Design review of the part built by this model. Coordinates are the model's own, in mm. A direction names the side the tool comes from. Round coordinates to 2 decimals unless told otherwise and drop trailing zeros. Order: outer loops, then holes, each group sorted by start corner. A loop starts at its lowest first (then second) coordinate and runs counter-clockwise, first axis right, second up. Notation, with made-up numbers: M 60,76.5 L 103,76.5 A29 cw 103,97.5 Z; hole C -20,40 d1. An arc over 180 degrees is marked long. Use a Markdown table: item, result. Add a question column.
(1) Machinability: for faces 4 (the face through (22, -17.2, 1)), 5 (the face through (-13.417, -29.187, 1.014)), 6 (the face through (17, -22.1, 1)), 7 (the face through (28.733, 5.205, 1.014)), 8 (the face through (-25, 25, 1)), which of the approach directions +Z, -Z, +X, -X, +Y, -Y give a long, thin tool a straight path to every point of the face, cutting with its end or side? Answer none if there is none.
(2) Take a section at C-C (x = -28.5). Write out the cut boundary in (y, z).
(3) Take a section at B-B (z = 1.3). Write out the cut boundary in (x, y), then the cut area to 3 significant figures.
(4) Take a section at A-A (y = 21.73). Write out the cut boundary in (x, z).
(5) Take a section at D-D (y = -8.6). Write out the cut boundary in (x, z), then the cut area to 3 significant figures.
(6) The part is to be moulded in two halves that separate along Y. For faces 1 (the face through (-28.733, 5.205, 1.014)), 2 (the face through (-17, -22.1, 1)), 3 (the face through (32.364, -4, 1)), say which applies: released by +Y, released by -Y, zero draft, split by the parting line, or undercut.
(7) To check wall thickness, follow probe 1 along X at (y, z) = (15.5, 1.9); probe 2 along Y at (x, z) = (-28.5, 0.95); probe 3 along Y at (x, z) = (19.5, 0.3). State the ranges of each line that lie inside material, in increasing order. Write a range as from..to.
```python
from build123d import *

# Parameters (mm, degrees)
EXTRUDE1_DEPTH  = 2
SKETCH4_R       = 1.5
EXTRUDE3_DEPTH  = 2
EXTRUDE5_DEPTH  = 2
FILLET2_R       = 3
SKETCH7_R       = 1.5
EXTRUDE6_DEPTH  = 2
EXTRUDE7_DEPTH  = 2
EXTRUDE8_DEPTH  = 2
EXTRUDE9_DEPTH  = 2
EXTRUDE10_DEPTH = 2
EXTRUDE11_DEPTH = 2
SKETCH13_W      = 52.444820885
SKETCH13_H      = 24.426279397
EXTRUDE12_DEPTH = 2
SKETCH14_R      = 1.5
EXTRUDE13_DEPTH = 2


with BuildPart() as part:
    # Sketch1 → Extrude1 (new body)
    with BuildSketch(Plane.XY):
        Polygon((-15, 13.5), (-15, 38.5), (15, 38.5), (15, 13.5), (26.811651575, -4.688348425), (15, -16.5), (15, -26.5), (7.928932188, -33.571067812), (7.928932188, -52.571067812), (-7.928932188, -52.571067812), (-7.928932188, -33.571067812), (-15, -26.5), (-15, -16.5), (-26.811651575, -4.688348425), align=None)
    extrude(amount=EXTRUDE1_DEPTH)

    # Sketch4 → Extrude3 (add)
    with BuildSketch(Plane.XY.offset(2)):
        Polygon((-26.811651575, -4.688348425), (-32.363678884, -6.963209468), (-30.088817841, -12.515236776), (-22.212122569, -9.287877431), align=None)
        with Locations((-28.5, -8.6)):
            Circle(SKETCH4_R, mode=Mode.SUBTRACT)
    extrude3 = extrude(amount=-EXTRUDE3_DEPTH)

    # Mirror1: Extrude3 across plane
    add(extrude3.mirror(Plane(origin=(0, 0, 0), x_dir=(0, 0, 1), z_dir=(1, 0, 0))))

    # Sketch6 → Extrude5 (add)
    with BuildSketch(Plane.XY.offset(2)):
        Polygon((0, -44.571067812), (-7.928932188, -44.571067812), (-18, -54.642135624), (18, -54.642135624), (7.928932188, -44.571067812), align=None)
    extrude(amount=-EXTRUDE5_DEPTH)

    # Fillet2
    fillet2_edges = [part.edges().sort_by_distance(p)[0] for p in [
        (18, -54.642135624, 1),
        (-18, -54.642135624, 1),
    ]]
    fillet(fillet2_edges, radius=FILLET2_R)

    # Sketch7 → Extrude6 (cut)
    with BuildSketch(Plane.XY.offset(2)):
        with Locations((-11, -52.002135624)):
            Circle(SKETCH7_R)
    extrude6 = extrude(amount=-EXTRUDE6_DEPTH, mode=Mode.SUBTRACT)

    # Mirror4: Extrude6 across plane
    add(extrude6.mirror(Plane(origin=(0, 0, 0), x_dir=(0, 0, 1), z_dir=(1, 0, 0))), mode=Mode.SUBTRACT)

    # Sketch8 → Extrude7 (add)
    with BuildSketch(Plane.XY.offset(2)):
        Polygon((-26.811651575, -4.688348425), (-32.363678884, -6.963209468), (-32.363678884, -0.385171544), (-15, 26.352549211), (-15, 13.5), align=None)
    extrude7 = extrude(amount=-EXTRUDE7_DEPTH)

    # Sketch9 → Extrude8 (add)
    with BuildSketch(Plane.XY.offset(2)):
        Polygon((-22.212122569, -9.287877431), (-25.22165278, -10.520987907), (-15, -20.742640687), (-15, -16.5), align=None)
    extrude8 = extrude(amount=-EXTRUDE8_DEPTH)

    # Sketch10 → Extrude9 (add)
    with BuildSketch(Plane.XY.offset(2)):
        Polygon((-25.22165278, -10.520987907), (-30.088817841, -12.515236776), (-23.702612277, -18.90144234), (-20.271905312, -15.470735375), align=None)
    extrude9 = extrude(amount=-EXTRUDE9_DEPTH)

    # Sketch11 → Extrude10 (add)
    with BuildSketch(Plane.XY.offset(2)):
        Polygon((-15.322157844, -20.420482843), (-18.752864809, -23.851189808), (-7.928932188, -34.675122429), (-7.928932188, -33.571067812), (-15, -26.5), (-15, -20.742640687), align=None)
    extrude10 = extrude(amount=-EXTRUDE10_DEPTH)

    # Sketch12 → Extrude11 (add)
    with BuildSketch(Plane.XY.offset(2)):
        Polygon((-25, 10.953899573), (-25, 38.5), (-15, 38.5), (-15, 26.352549211), align=None)
    extrude11 = extrude(amount=-EXTRUDE11_DEPTH)

    # Mirror5: Extrude7, Extrude8, Extrude9, Extrude10 across plane
    add(extrude7.mirror(Plane(origin=(0, 0, 0), x_dir=(0, 0, 1), z_dir=(1, 0, 0))))
    add(extrude8.mirror(Plane(origin=(0, 0, 0), x_dir=(0, 0, 1), z_dir=(1, 0, 0))))
    add(extrude9.mirror(Plane(origin=(0, 0, 0), x_dir=(0, 0, 1), z_dir=(1, 0, 0))))
    add(extrude10.mirror(Plane(origin=(0, 0, 0), x_dir=(0, 0, 1), z_dir=(1, 0, 0))))

    # Mirror6: Extrude11 across plane
    add(extrude11.mirror(Plane(origin=(0, 0, 0), x_dir=(0, 0, 1), z_dir=(1, 0, 0))))

    # Sketch13 → Extrude12 (cut)
    with BuildSketch(Plane(origin=(0, 0, 0), x_dir=(-1, 0, 0), z_dir=(0, 0, -1))):
        with Locations((1.088066824, -46.888262128)):
            Rectangle(SKETCH13_W, SKETCH13_H)
    extrude(amount=-EXTRUDE12_DEPTH, mode=Mode.SUBTRACT)

    # Sketch14 → Extrude13 (cut)
    with BuildSketch(Plane.XY.offset(2)):
        with Locations((-20, 21.73)):
            Circle(SKETCH14_R)
        with Locations((20, 21.73)):
            Circle(SKETCH14_R)
    extrude(amount=-EXTRUDE13_DEPTH, mode=Mode.SUBTRACT)


solid = part.part
```
Verdict:
| question | item | result |
|---|---|---|
| 1 | face 4 | +Z, -Z, -Y |
| 1 | face 5 | +Z, -Z, -X, -Y |
| 1 | face 6 | +Z, -Z, +X |
| 1 | face 7 | +Z, -Z, +X, +Y |
| 1 | face 8 | +Z, -Z, -X, +Y |
| 2 | outline | M -14.1,0 L -10.1,0 L -10.1,2 L -14.1,2 Z; M -7.1,0 L 5.56,0 L 5.56,2 L -7.1,2 Z |
| 3 | outline | M -32.36,-6.96 L -30.09,-12.52 L -23.7,-18.9 L -20.27,-15.47 L -15.32,-20.42 L -18.75,-23.85 L -7.93,-34.68 L 7.93,-34.68 L 18.75,-23.85 L 15.32,-20.42 L 20.27,-15.47 L 23.7,-18.9 L 30.09,-12.52 L 32.36,-6.96 L 32.36,-0.39 L 25,10.95 L 25,38.5 L -25,38.5 L -25,10.95 L -32.36,-0.39 Z; hole C -28.5,-8.6 d3; hole C -20,21.73 d3; hole C 20,21.73 d3; hole C 28.5,-8.6 d3 |
| 3 | area | 3,550 mm^2 |
| 4 | outline | M -25,0 L -21.5,0 L -21.5,2 L -25,2 Z; M -18.5,0 L 18.5,0 L 18.5,2 L -18.5,2 Z; M 21.5,0 L 25,0 L 25,2 L 21.5,2 Z |
| 5 | outline | M -31.69,0 L -30,0 L -30,2 L -31.69,2 Z; M -27,0 L 27,0 L 27,2 L -27,2 Z; M 30,0 L 31.69,0 L 31.69,2 L 30,2 Z |
| 5 | area | 115 mm^2 |
| 6 | face 1 | released by +Y |
| 6 | face 2 | undercut |
| 6 | face 3 | zero draft |
| 7 | probe 1 | x = -25..25 |
| 7 | probe 2 | y = -14.1..-10.1, -7.1..5.56 |
| 7 | probe 3 | y = -16.24..20.32, 23.14..38.5 |
